```python
from build123d import *

# Parameters (mm, degrees)
SKETCH1_W            = 70
SKETCH1_H            = 50
BOSS_EXTRUDE1_DEPTH  = 50
CUT_EXTRUDE1_DEPTH   = 50
CUT_EXTRUDE2_DEPTH   = 20
CUT_EXTRUDE3_DEPTH   = 20
CUT_EXTRUDE4_DEPTH   = 5
BOSS_EXTRUDE2_DEPTH  = 25
CUT_EXTRUDE5_DEPTH   = 25
BOSS_EXTRUDE3_DEPTH  = 30
BOSS_EXTRUDE4_DEPTH  = 50
CUT_EXTRUDE7_DEPTH   = 15
CUT_EXTRUDE8_DEPTH   = 15
BOSS_EXTRUDE5_DEPTH  = 15
CUT_EXTRUDE12_DEPTH  = 15
CUT_EXTRUDE13_DEPTH  = 15
BOSS_EXTRUDE6_DEPTH  = 15
SKETCH22_W           = 70
SKETCH22_H           = 50
CUT_EXTRUDE15_DEPTH  = 15
BOSS_EXTRUDE11_DEPTH = 15
CUT_EXTRUDE18_DEPTH  = 15
CUT_EXTRUDE19_DEPTH  = 15
BOSS_EXTRUDE14_DEPTH = 15
BOSS_EXTRUDE17_DEPTH = 25
BOSS_EXTRUDE18_DEPTH = 25


with BuildPart() as part:
    # Sketch1 → Boss-Extrude1 (new body)
    with BuildSketch(Plane.XY):
        with Locations((35, 25)):
            Rectangle(SKETCH1_W, SKETCH1_H)
    extrude(amount=BOSS_EXTRUDE1_DEPTH)

    # Sketch2 → Cut-Extrude1 (cut)
    with BuildSketch(Plane.XZ):
        Polygon((0, 30), (20, 50), (0, 50), align=None)
    extrude(amount=-CUT_EXTRUDE1_DEPTH, mode=Mode.SUBTRACT)

    # Sketch3 → Cut-Extrude2 (cut)
    with BuildSketch(Plane.XY.offset(50)):
        Polygon((60, 0), (60, 50), (40, 50), (20, 30), (20, 0), align=None)
    extrude(amount=-CUT_EXTRUDE2_DEPTH, mode=Mode.SUBTRACT)

    # Sketch4 → Cut-Extrude3 (cut)
    with BuildSketch(Plane(origin=(0, 50, 0), x_dir=(1, 0, 0), z_dir=(0, 1, 0))):
        Polygon((40, -30), (20, -50), (0, -30), (0, 0), (40, -20), align=None)
    extrude(amount=-CUT_EXTRUDE3_DEPTH, mode=Mode.SUBTRACT)

    # Sketch5 → Cut-Extrude4 (cut)
    with BuildSketch(Plane(origin=(0, 30, 0), x_dir=(1, 0, 0), z_dir=(0, 1, 0))):
        Polygon((0, 0), (0, -30), (20, -50), (20, -30), (40, -30), (40, -20), align=None)
    extrude(amount=-CUT_EXTRUDE4_DEPTH, mode=Mode.SUBTRACT)

    # Sketch6 → Boss-Extrude2 (add)
    with BuildSketch(Plane(origin=(0, 25, 0), x_dir=(1, 0, 0), z_dir=(0, 1, 0))):
        Polygon((20, -10), (20, -30), (40, -30), (40, -20), align=None)
    extrude(amount=BOSS_EXTRUDE2_DEPTH)

    # Sketch7 → Cut-Extrude5 (cut)
    with BuildSketch(Plane(origin=(0, 50, 0), x_dir=(1, 0, 0), z_dir=(0, 1, 0))):
        Polygon((20, -50), (40, -50), (40, -30), align=None)
    extrude(amount=-CUT_EXTRUDE5_DEPTH, mode=Mode.SUBTRACT)

    # Sketch8 → Boss-Extrude3 (add)
    with BuildSketch(Plane.XZ):
        Polygon((20, 50), (20, 40), (40, 30), (60, 30), (60, 50), align=None)
    extrude(amount=-BOSS_EXTRUDE3_DEPTH)

    # Sketch9 → Boss-Extrude4 (add)
    with BuildSketch(Plane(origin=(0, 50, 0), x_dir=(1, 0, 0), z_dir=(0, 1, 0))):
        Polygon((20, -40), (40, -30), (20, -30), align=None)
    extrude(amount=-BOSS_EXTRUDE4_DEPTH)

    # Sketch10 → Cut-Extrude7 (cut)
    with BuildSketch(Plane(origin=(0, 50, 0), x_dir=(1, 0, 0), z_dir=(0, 1, 0))):
        Polygon((20, -40), (40, -30), (40, -20), (20, -10), align=None)
    extrude(amount=-CUT_EXTRUDE7_DEPTH, mode=Mode.SUBTRACT)

    # Sketch11 → Cut-Extrude8 (cut)
    with BuildSketch(Plane(origin=(0, 17.24137931, 43.103448276), x_dir=(1, 0, 0), z_dir=(0, 0.371390676, 0.928476691))):
        Polygon((60, 35.282114254), (60, -18.569533818), (20, -18.569533818), (20, 4.642383454), (40, 35.282114254), align=None)
    extrude(amount=CUT_EXTRUDE8_DEPTH, mode=Mode.SUBTRACT)

    # Sketch12 → Boss-Extrude5 (add)
    with BuildSketch(Plane(origin=(0, 17.24137931, 43.103448276), x_dir=(1, 0, 0), z_dir=(0, 0.371390676, 0.928476691))):
        Polygon((40, 35.282114254), (60, 35.282114254), (60, -18.569533818), (20, -18.569533818), (20, 4.642383454), align=None)
    extrude(amount=-BOSS_EXTRUDE5_DEPTH)

    # Sketch13 → Cut-Extrude12 (cut)
    with BuildSketch(Plane(origin=(11.899549259, -7.211848036, 2.884739214), x_dir=(0.173608446, -0.10521724, -0.979177941), z_dir=(0.837390852, -0.507509607, 0.203003843))):
        Polygon((-48.11715912, 31.745980111), (-48.11715912, 37.592580529), (-35.861981078, 39.10036734), (-39.313151906, 28.797022071), align=None)
    extrude(amount=-CUT_EXTRUDE12_DEPTH, mode=Mode.SUBTRACT)

    # Sketch15 → Cut-Extrude13 (cut)
    with BuildSketch(Plane(origin=(0, 17.24137931, 43.103448276), x_dir=(1, 0, 0), z_dir=(0, 0.371390676, 0.928476691))):
        Polygon((40, 35.282114254), (20, 35.282114254), (20, -18.569533818), align=None)
    extrude(amount=CUT_EXTRUDE13_DEPTH, mode=Mode.SUBTRACT)

    # Sketch16 → Boss-Extrude6 (add)
    with BuildSketch(Plane(origin=(0, 17.24137931, 43.103448276), x_dir=(1, 0, 0), z_dir=(0, 0.371390676, 0.928476691))):
        Polygon((25.939393939, 13.741455025), (28, 19.126619832), (24, 13.741455025), align=None)
        Polygon((28, 19.126619832), (25.939393939, 13.741455025), (29.454545455, 19.126619832), align=None)
    extrude(amount=-BOSS_EXTRUDE6_DEPTH)

    # Sketch22 → Cut-Extrude15 (cut)
    with BuildSketch(Plane(origin=(0, 0, 0), x_dir=(-1, 0, 0), z_dir=(0, -1, 0))):
        with Locations((-35, -25)):
            Rectangle(SKETCH22_W, SKETCH22_H)
    extrude(amount=CUT_EXTRUDE15_DEPTH, mode=Mode.SUBTRACT)

    # Sketch28 → Boss-Extrude11 (add)
    with BuildSketch(Plane(origin=(-9.6, 12.8, 0), x_dir=(0.8, 0.6, 0), z_dir=(-0.6, 0.8, 0))):
        Polygon((37, -36), (62, -30), (62, -20), (37, -10), align=None)
    extrude(amount=-BOSS_EXTRUDE11_DEPTH)

    # Sketch29 → Cut-Extrude18 (cut)
    with BuildSketch(Plane(origin=(0, 0, 0), x_dir=(0, 0, -1), z_dir=(0.780868809, -0.624695048, 0))):
        Polygon((-40, 32.015621187), (-30, 64.031242374), (-20, 64.031242374), (-10, 32.015621187), align=None)
    extrude(amount=-CUT_EXTRUDE18_DEPTH, mode=Mode.SUBTRACT)

    # Sketch30 → Cut-Extrude19 (cut)
    with BuildSketch(Plane(origin=(0, 0, 0), x_dir=(0.894427191, 0, 0.447213595), z_dir=(-0.447213595, 0, 0.894427191))):
        Polygon((0, 50), (44.72135955, 50), (22.360679775, 25), (0, 25), align=None)
    extrude(amount=CUT_EXTRUDE19_DEPTH, mode=Mode.SUBTRACT)

    # Sketch32 → Boss-Extrude14 (add)
    with BuildSketch(Plane(origin=(0, 17.24137931, 43.103448276), x_dir=(1, 0, 0), z_dir=(0, 0.371390676, 0.928476691))):
        Polygon((28, 19.126619832), (40, 35.282114254), (29.454545455, 19.126619832), align=None)
    extrude(amount=-BOSS_EXTRUDE14_DEPTH)

    # Sketch34 → Boss-Extrude17 (add)
    with BuildSketch(Plane(origin=(0, 25, 0), x_dir=(1, 0, 0), z_dir=(0, 1, 0))):
        Polygon((14.310344828, -40), (20, -40), (20, -50), align=None)
    extrude(amount=-BOSS_EXTRUDE17_DEPTH)

    # Sketch35 → Boss-Extrude18 (add)
    with BuildSketch(Plane(origin=(0, 0, 0), x_dir=(0, 0, 1), z_dir=(-0.780868809, 0.624695048, 0))):
        Polygon((30, 64.031242374), (40, 32.015621187), (10, 32.015621187), (20, 64.031242374), align=None)
    extrude(amount=-BOSS_EXTRUDE18_DEPTH)


solid = part.part
```
The model under review builds one solid part; all positions refer to its coordinate system, in mm. A direction names the side the tool comes from. Give positions to 0.01 mm unless a question says otherwise; leave off trailing zeros. Loops run counter-clockwise (first coordinate to the right, second up) from the corner with the lowest first, then second, coordinate; pieces in that order, holes last. Notation, with made-up numbers: (76, 86.5) - (101, 86.5) arc R11 cw to (101, 91.5) - close; hole circle Ø4 at (28, -7.5). An arc over 180 degrees is marked (long way). Answer as a JSON object with one key per item and string values.
Q1. Add section C-C on z = 47. State the section outline as (x, y) points.
Worked out:
{"outline": "(17, 0) - (70, 0) - (70, 50) - (60, 50) - (60, 7.5) - (20, 7.5) - (20, 25) - (17, 25) - close"}
Q2. For faces 1 (the flat face through (50, 50, 14)), 2 (the flat face through (10, 25, 25)), 3 (the flat face through (60, 36, 45)), list the 3-axis set-ups (+Z, -Z, +X, -X, +Y, -Y) from which the entire face can be reached by the end or side of a thin tool; tool diameter is ignored.
Worked out:
{"face 1": "+Z, -Z, +X, -X, +Y", "face 2": "+Z, -X, +Y", "face 3": "+Z, +Y"}
Q3. Add section B-B on y = 20.5. State the section outline as (x, z) points, plus the area to 3 significant figures.
Worked out:
{"outline": "(0, 0) - (70, 0) - (70, 50) - (60, 50) - (60, 41.8) - (20, 41.8) - (20, 50) - (0, 30) - close", "area": "2,970 mm^2"}
Q4. To check wall thickness, follow line 1 along Y through (x, z) = (12, 23); line 2 along X through (y, z) = (40, 43); line 3 along X through (y, z) = (16, 45). State the ranges of each line that lie inside material, in increasing order.
Worked out:
{"line 1": "y = 0 to 25", "line 2": "x = 60 to 70", "line 3": "x = 15 to 20, 60 to 70"}
Q5. Add section A-A on x = 32. State the section outline as (y, z) points.
Worked out:
{"outline": "(0, 0) - (50, 0) - (50, 16) - (40, 16) - (40, 34) - (0, 50) - close"}
Q6. Mouldability with a two-part tool opening along X and no side actions: class faces 4 (the flat face through (35, 0, 25)), 5 (the flat face through (28, 35, 25)), 6 (the flat face through (20, 16, 47)), 7 (the flat face through (70, 25, 25)) as +X half, -X half, draft (parallel to the pull), parting line (faces both ways), or undercut.
Worked out:
{"face 4": "draft", "face 5": "-X half", "face 6": "undercut", "face 7": "+X half"}
Q7. Insertion check: pin 1 (16 mm diameter, centred on y = 23, z = 40, fed in from -X); pin 2 (2 mm diameter, centred on x = 21, z = 12, fed in from +Y); pin 3 (2 mm diameter, centred on x = 40.5, y = 25, fed in from +Z). Each pin has a flat end and moves straight along its axis. Give the tip position at first contact, or say it passes through.
Worked out:
{"pin 1": "stops at x = 2", "pin 2": "stops at y = 27.5", "pin 3": "stops at z = 40.4"}
Q8. Add section D-D on x = 18. State the section outline as (y, z) points.
Worked out:
{"outline": "(0, 0) - (50, 0) - (50, 9) - (25, 9) - (25, 48) - (0, 48) - close"}
